Geometry: final body of the model. Coordinates: model frame, mm. Face numbers are marked on the shaded views. A direction names the side the tool comes from. Give positions to 0.01 mm unless a question says otherwise; leave off trailing zeros. Write each loop counter-clockwise with the first axis right and the second up, starting at its lowest first coordinate (ties: lowest second). Pieces come first, ordered by that corner, then holes.
from build123d import *

# Parameters (mm, degrees)
F0_W     = 36.951749
F0_H     = 20.582954
F1_DEPTH = 73.328344
F4_D     = 6.35
F5_W     = 10.310262
F5_H     = 10.642964
F3_DEPTH = 25.4


with BuildPart() as f1:
    # F0 (on Front) → F1 (new body)
    with BuildSketch(Plane.XZ):
        with Locations((31.52898, 21.655689)):
            Rectangle(F0_W, F0_H)
    extrude(amount=F1_DEPTH)

    # F4 (through all)
    with Locations(Plane.XY.offset(31.947166)):
        with Locations((31.054407, -35.539657)):
            Hole(F4_D / 2)

    # F5 (on face) → F3 (cut)
    with BuildSketch(Plane.XY.offset(31.947166)):
        with Locations((30.807659, -52.12252)):
            Rectangle(F5_W, F5_H)
    extrude(amount=-F3_DEPTH, mode=Mode.SUBTRACT)


solid = f1.part
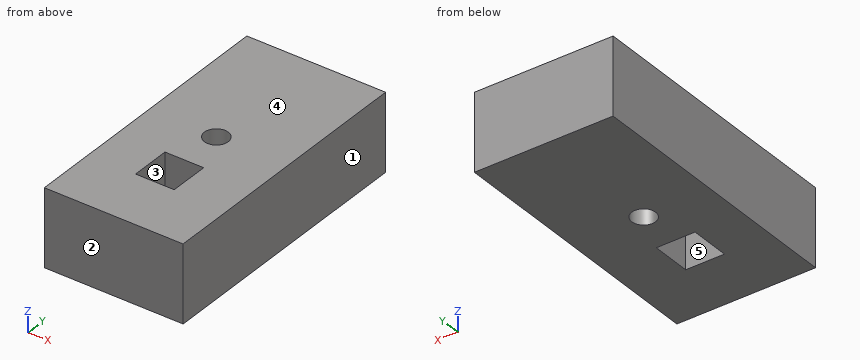
Q1. Access query for the marked faces 4 and 5. Directions: +Z, -Z, +X, -X, +Y, -Y. A direction counts if a zero-diameter tool reaches every point of the face in a straight line with its end or side. Return the directions, or none.
Filled sheet:
face 4: +Z, +X, -X, +Y, -Y
face 5: +Z, -Z
Q2. Pull-direction query (Y, two-part tool) for the marked faces 1, 2 and 3; classes: released by +Y, released by -Y, zero draft, split by the parting line, or undercut.
Filled sheet:
face 1: zero draft
face 2: released by -Y
face 3: undercut
Q3. Ray query, line 1 along X through (y, z) = (-54, 15.25); line 2 along Y through (x, z) = (31, 19.25). Return the intervals inside material, ascending.
Filled sheet:
line 1: x = 13.05 to 25.65, 35.96 to 50
line 2: y = -73.33 to -57.44, -46.8 to -38.71, -32.37 to 0
Q4. Section B-B on x = 31.5. Output: boundary loops of the cut face in (y, z).
Filled sheet:
outline: (-73.33, 11.36) - (-57.44, 11.36) - (-57.44, 31.95) - (-73.33, 31.95) - close; (-46.8, 11.36) - (-38.68, 11.36) - (-38.68, 31.95) - (-46.8, 31.95) - close; (-32.4, 11.36) - (0, 11.36) - (0, 31.95) - (-32.4, 31.95) - close
Q5. Section A-A on y = -53. Output: boundary loops of the cut face in (x, z), plus the area to 3 significant figures.
Filled sheet:
outline: (13.05, 11.36) - (25.65, 11.36) - (25.65, 31.95) - (13.05, 31.95) - close; (35.96, 11.36) - (50, 11.36) - (50, 31.95) - (35.96, 31.95) - close
area: 548 mm2
Q6. Section C-C on z = 17.25. Output: boundary loops of the cut face in (x, y) (3 decimals).
Filled sheet:
outline: (13.053, -73.328) - (50.005, -73.328) - (50.005, 0) - (13.053, 0) - close; hole (25.653, -57.444) - (35.963, -57.444) - (35.963, -46.801) - (25.653, -46.801) - close; hole circle Ø6.35 at (31.054, -35.54)
